CAD build for the part. Positions are in the model's coordinates, mm. Round coordinates to 2 decimals unless told otherwise and drop trailing zeros. Loops run counter-clockwise (first coordinate to the right, second up) from the corner with the lowest first, then second, coordinate; pieces in that order, holes last.
from build123d import *

# Parameters (mm, degrees)
EXTRUSION1_DEPTH = 245
CONG_1_R         = 2
ESQUISSE2_R      = 2
EXTRUSION2_DEPTH = 75


with BuildPart() as part:
    # Esquisse1 → Extrusion1 (new body)
    with BuildSketch(Plane(origin=(0, 0, 0), x_dir=(1, 0, 0), z_dir=(0, 1, 0))):
        with BuildLine():
            Line((0, 0), (0, 33))
            ThreePointArc((0, 33), (16.5, 49.5), (33, 33))
            Line((33, 33), (33, 0))
            ThreePointArc((33, 0), (16.5, -16.5), (0, 0))
        make_face()
    extrude(amount=EXTRUSION1_DEPTH)

    # Congé1
    cong_1_edges = [part.edges().sort_by_distance(p)[0] for p in [
        (16.5, 245, -49.5),
        (0, 245, -16.5),
        (16.5, 245, 16.5),
        (0, 0, -16.5),
        (16.5, 0, -49.5),
        (33, 0, -16.5),
        (16.5, 0, 16.5),
        (33, 245, -16.5),
    ]]
    fillet(cong_1_edges, radius=CONG_1_R)

    # Esquisse2 → Extrusion2 (add)
    with BuildSketch(Plane(origin=(0, 245, 0), x_dir=(1, 0, 0), z_dir=(0, 1, 0))):
        with Locations((16.5, 18.6)):
            Circle(ESQUISSE2_R)
        with Locations((16.5, 14.4)):
            Circle(ESQUISSE2_R)
    extrude(amount=EXTRUSION2_DEPTH)


solid = part.part
Item 1: Cut at B-B (y = 265). List the corners of the cut face in (x, z), plus the area to 3 significant figures.
Verdict:
outline: circle Ø4 at (16.5, -18.6); circle Ø4 at (16.5, -14.4)
area: 25.1 mm2
Item 2: Flat gauge pins, fed straight in: P1, Ø14.5, axis at x = 15, z = -30, coming from the +Y side; P2, Ø5, axis at x = 18.5, y = 269, coming from the -Z side; P3, Ø3, axis at y = 60, z = -36, coming from the -X side. Where does each tip first touch, or does it go through?
Verdict:
P1: stops at y = 245
P2: stops at z = -20.6
P3: stops at x = 0.07
Item 3: Cut at C-C (y = 48). List the corners of the cut face in (x, z), plus the area to 3 significant figures.
Verdict:
outline: (0, -33) arc R16.5 ccw to (33, -33) - (33, 0) arc R16.5 ccw to (0, 0) - close
area: 1,940 mm2
Item 4: Cut at A-A (z = -9). List the corners of the cut face in (x, y), plus the area to 3 significant figures.
Verdict:
outline: (0, 2) arc R2 ccw to (2, 0) - (31, 0) arc R2 ccw to (33, 2) - (33, 243) arc R2 ccw to (31, 245) - (2, 245) arc R2 ccw to (0, 243) - close
area: 8,080 mm2
Item 5: Wall check: L1, parallel to Y at x = 3.5, z = 7.5; L2, parallel to Y at x = 11.5, z = -32.5; L3, parallel to Z at x = 17, y = 298. Give the ranges that are in metal, low to high.
Verdict:
L1: y = 0.07 to 244.93
L2: y = 0 to 245
L3: z = -20.54 to -16.66, -16.34 to -12.46
